```python
from build123d import *

# Parameters (mm, degrees)
F1_DEPTH  = 95
F2_W      = 35
F2_H      = 25
F3_DEPTH  = 2
F4_W      = 92.7402563393
F4_H      = 113.4333282709
F5_DEPTH  = 45
F7_DEPTH  = 92.7402563393
F10_DEPTH = 47.8


with BuildPart() as f1:
    # F0 (on Top) → F1 (new body)
    with BuildSketch(Plane.XY):
        Polygon((-21.8103982317, -11.2208545208), (13.1896017683, -11.2208545208), (13.1896017683, 13.7791454792), (3.1896017683, 13.7791454792), (3.1896017683, 8.7791454792), (8.1896017683, 8.7791454792), (8.1896017683, -6.2208545208), (-16.8103982317, -6.2208545208), (-16.8103982317, 8.7791454792), (-11.8103982317, 8.7791454792), (-11.8103982317, 13.7791454792), (-21.8103982317, 13.7791454792), align=None)
    extrude(amount=F1_DEPTH)

    # F2 (on face) → F3 (join)
    with BuildSketch(Plane(origin=(0, 0, 0), x_dir=(1, 0, 0), z_dir=(0, 0, -1))):
        with Locations((-4.3103982317, -1.2791454792)):
            Rectangle(F2_W, F2_H)
    extrude(amount=F3_DEPTH)

    # F4 (on face) → F5 (join)
    with BuildSketch(Plane(origin=(0, 0, -2), x_dir=(1, 0, 0), z_dir=(0, 0, -1))):
        with Locations((-4.7465320677, -45.4958096147)):
            Rectangle(F4_W, F4_H)
    extrude(amount=F5_DEPTH)

    # F6 (on face) → F7 (cut, through all)
    with BuildSketch(Plane(origin=(-51.1166602373, 0, 0), x_dir=(0, -1, 0), z_dir=(-1, 0, 0))):
        Polygon((-102.2124737501, -28.7785492837), (-13.7791454792, -2), (-102.2124737501, -2), align=None)
    extrude(amount=-F7_DEPTH, mode=Mode.SUBTRACT)

    # F9 (on 3pt) → F10 (cut)
    with BuildSketch(Plane(origin=(-23.1632746384, -5.9843875324, 0), x_dir=(-0.2501432541, 0.9682088372, 0), z_dir=(0.9682088372, 0.2501432541, 0))):
        Polygon((111.7495080876, 32.3685184121), (-5.4084065206, -2), (-6.0562286526, -47), (111.7495080876, -47), align=None)
    extrude(amount=-F10_DEPTH, mode=Mode.SUBTRACT)


solid = f1.part
```
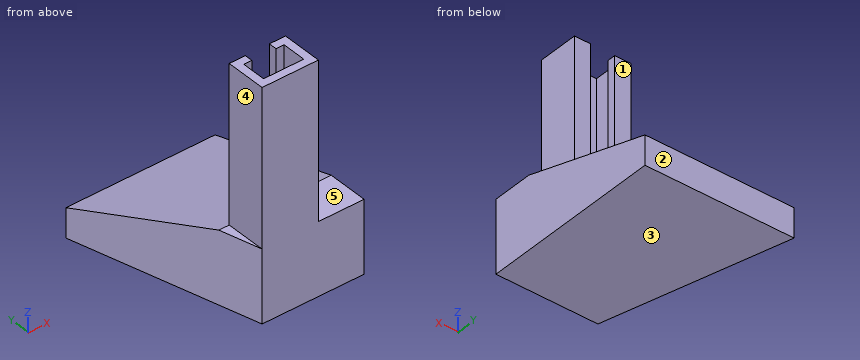
Geometry: final body of the model. Coordinates: model frame, mm. Face numbers are marked on the shaded views. A direction names the side the tool comes from. Coordinates: 2 decimals unless noted, no trailing zeros. Write each loop counter-clockwise with the first axis right and the second up, starting at its lowest first coordinate (ties: lowest second). Pieces come first, ordered by that corner, then holes. Notation, with made-up numbers: M 50,-39.5 L 67,-39.5 A34 cw 67,-6.5 Z; hole C 40.25,83 d4. An arc over 180 degrees is marked long. Use CSV: the item, a comma, the result in double quotes. Start each with the question number.
1. Cut plane C-C on y = 2. Return the cut outline in (x, z).
2. Reachability of the marked faces 1, 2, 3, 4 and 5 from +Z, -Z, +X, -X, +Y, -Y: full face, straight path, thin tool, end or side. Return the list, or none.
3. Cut plane B-B on z = 39. Return the cut outline in (x, y), plus the area to 3 significant figures.
4. Cut plane A-A on x = 5.5. Return the cut outline in (y, z), plus the area to 3 significant figures.
5. First-contact query: P1, Ø5.5, axis at y = 11.5, z = 53.5, coming from the +X side; P2, Ø2, axis at y = 50, z = -30, coming from the -X side; P3, Ø10.5, axis at x = -7, z = 51, coming from the +Y side. Flat tips, straight axial feed; report the tip coordinate or a pass-through.
6. Cut plane D-D on x = 22. Return the cut outline in (y, z).
7. Ray query, probe 1 along X at (y, z) = (4, 47); probe 2 along Y at (x, z) = (-17, -1.5); probe 3 along Z at (x, y) = (-22.5, 9). Return the intervals inside material, ascending.
Entries:
1,outline,"M -25.23,-47 L 41.62,-47 L 41.62,-2 L 13.19,-2 L 13.19,95 L 8.19,95 L 8.19,0 L -16.81,0 L -16.81,95 L -21.81,95 L -21.81,-2 L -25.23,-2 Z"
2,face 1,"+Z, +X, -X, +Y"
2,face 2,"+Z, -Z, +X, -X, +Y"
2,face 3,"-Z, +X, -X, +Y, -Y"
2,face 4,"+Z, -X, +Y, -Y"
2,face 5,"+Z, +X, +Y, -Y"
3,outline,"M -21.81,-11.22 L 13.19,-11.22 L 13.19,13.78 L 3.19,13.78 L 3.19,8.78 L 8.19,8.78 L 8.19,-6.22 L -16.81,-6.22 L -16.81,8.78 L -11.81,8.78 L -11.81,13.78 L -21.81,13.78 Z"
3,area,"425 mm²"
4,outline,"M -11.22,-47 L 102.21,-47 L 102.21,-28.78 L 13.78,-2 L 13.78,95 L 8.78,95 L 8.78,0 L -6.22,0 L -6.22,95 L -11.22,95 Z"
4,area,"4,920 mm²"
5,P1,"x = 13.19"
5,P2,"x = -37.89"
5,P3,"y = 13.78"
6,outline,"M -11.22,-47 L 102.21,-47 L 102.21,-28.78 L 13.78,-2 L -11.22,-2 Z"
7,probe 1,"-21.81 to -16.81, 8.19 to 13.19"
7,probe 2,"-11.22 to 13.78"
7,probe 3,"-47 to -2"
